The figure shows three views and two pictorial views of one solid part (mm, origin at its lowest corner). Answer the questions. A direction names the side the tool comes from. Give positions to 0.01 mm unless a question says otherwise; leave off trailing zeros. Loops run counter-clockwise (first coordinate to the right, second up) from the corner with the lowest first, then second, coordinate; pieces in that order, holes last.
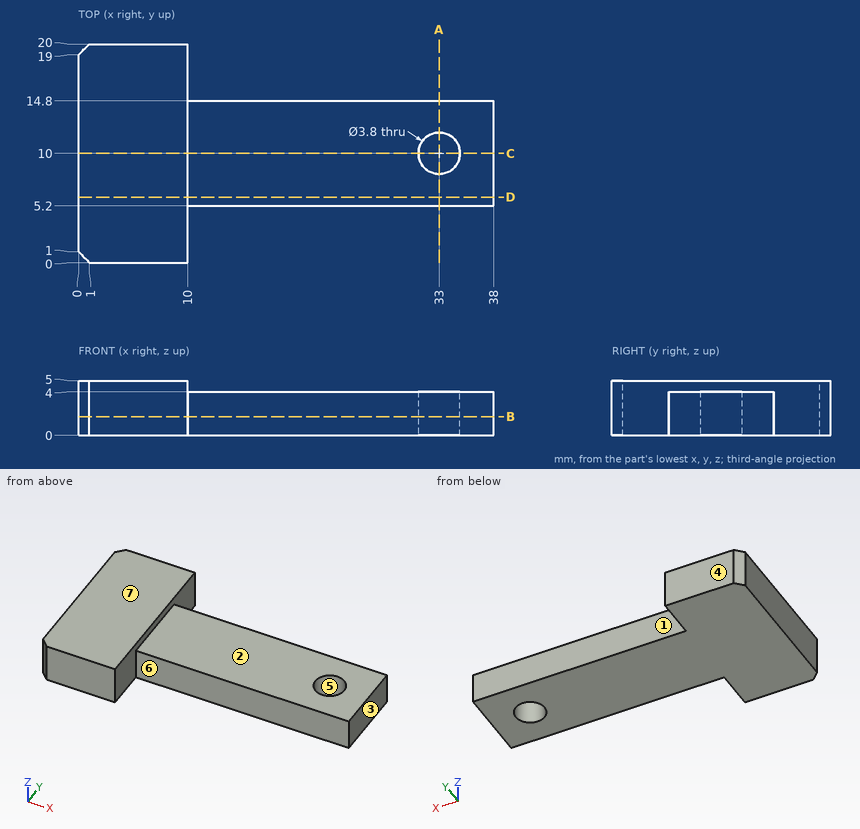
Q1. Section C-C on y = 10 is taken. Give the vertices of the cut face in (x, z), plus the area to 3 significant figures.
Q2. Consider line 1 along Y through (x, z) = (33, 2); line 2 along X through (y, z) = (10, 1); line 3 along Y through (x, z) = (19.5, 1.6). Determine where each line is inside the solid, lowest interval first.
Q3. Section B-B on z = 1.7 is taken. Give the vertices of the cut face in (x, y).
Q4. Section A-A on x = 33 is taken. Give the vertices of the cut face in (y, z).
Q5. Given pin 1 (7.5 mm diameter, centred on x = 28, y = 9.5, fed in from +Z); pin 2 (3 mm diameter, centred on x = 21, z = 2, fed in from +Y); pin 3 (1.2 mm diameter, centred on x = 29, z = 1.5, fed in from -Y), each flat-ended and moving along its own axis, determine where each tip first touches the part or whether it passes through.
Q6. Which of the six approach directions +Z, -Z, +X, -X, +Y, -Y give full straight-line access (tool end or side, diameter ignored) to the marked faces 1, 2 and 3?
Q7. Determine the mould class of the marked faces 4, 5, 6 and 7 for opening direction Y: +Y half, -Y half, draft (parallel to the pull), parting line (faces both ways), or undercut.
Q8. Section D-D on y = 6 is taken. Give the vertices of the cut face in (x, z).
Check result:
1. outline: (0, 0) - (31.1, 0) - (31.1, 4) - (10, 4) - (10, 5) - (0, 5) - close; (34.9, 0) - (38, 0) - (38, 4) - (34.9, 4) - close
1. area: 147 mm2
2. line 1: y = 5.2 to 8.1, 11.9 to 14.8
2. line 2: x = 0 to 31.1, 34.9 to 38
2. line 3: y = 5.2 to 14.8
3. outline: (0, 1) - (1, 0) - (10, 0) - (10, 5.2) - (38, 5.2) - (38, 14.8) - (10, 14.8) - (10, 20) - (1, 20) - (0, 19) - close; hole circle Ø3.8 at (33, 10)
4. outline: (5.2, 0) - (8.1, 0) - (8.1, 4) - (5.2, 4) - close; (11.9, 0) - (14.8, 0) - (14.8, 4) - (11.9, 4) - close
5. pin 1: stops at z = 4
5. pin 2: stops at y = 14.8
5. pin 3: stops at y = 5.2
6. face 1: +Z, -Z, +X, +Y
6. face 2: +Z, +X, +Y, -Y
6. face 3: +Z, -Z, +X, +Y, -Y
7. face 4: +Y half
7. face 5: undercut
7. face 6: -Y half
7. face 7: draft
8. outline: (0, 0) - (38, 0) - (38, 4) - (10, 4) - (10, 5) - (0, 5) - close
